Autodesk Inventor part; units mm, degrees
ref_plane "YZ Plane" through (0, 0, 0) normal (1, 0, 0) x (0, 1, 0)
ref_plane "XZ Plane" through (0, 0, 0) normal (0, 1, 0) x (-1, 0, 0)
ref_plane "XY Plane" through (0, 0, 0) normal (0, 0, 1) x (1, 0, 0)
sketch "Sketch1" plane through (0, 0, 0) normal (0, 0, 1) x (1, 0, 0)
  line L0 (0, -3.05) -> (0, 18.3) construction
  line L1 (-3.6, 0) -> (0.6, 0) construction
  line L2 (0, 5) -> (0, 15.25)
  line L3 (0, 15.25) -> (-3, 15.25)
  line L4 (-3, 15.25) -> (-3, 11)
  line L5 (-3, 11) -> (-1, 11)
  line L6 (-1, 11) -> (-1, 5)
  line L7 (-1, 5) -> (0, 5)
  point P0 (0, 0)
  dimension "d0" = 30.5
  dimension "d1" = 10
  dimension "d2" = 22
  dimension "d3" = 1
  dimension "d4" = 3
revolve "Revolution1" add sketch "Sketch1" angle 360 about axis through (-10, 0, 0) along (1, 0, 0)
sketch "Sketch2" plane through (-3, 0, 0) normal (-1, 0, 0) x (0, 0, 1)
  line L0 (0, -21.35) -> (0, 21.35)
  line L1 (-21.35, 0) -> (21.35, 0)
  point P0 (0, 0)
  point P1 (-13, 0)
  dimension "d6" = 13
hole "Hole1" at (-3, 0, -13) direction (1, 0, 0) diameter 2 end through all
mirror "Mirror1" about plane through (0, 0, 0) normal (0, 0, 1) of "Hole1"
properties part number "P119PorteLentilleSouple" material "ABS Plastic"
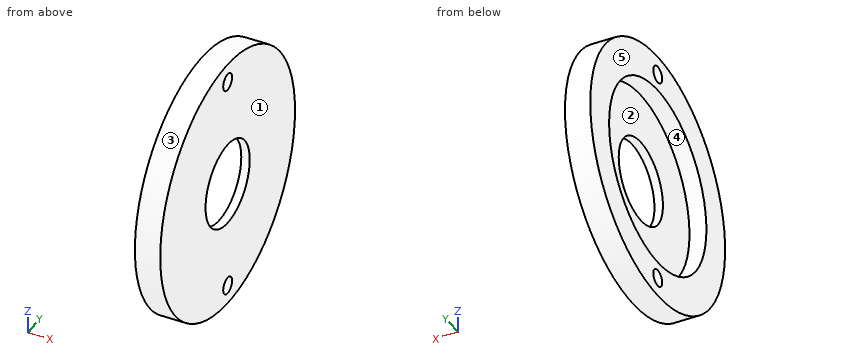
The listing builds one solid part. Answer for the finished solid, in the listing's coordinates (mm). Face numbers are marked on the shaded views. A direction names the side the tool comes from. Give positions to 0.01 mm unless a question says otherwise; leave off trailing zeros. Write each loop counter-clockwise with the first axis right and the second up, starting at its lowest first coordinate (ties: lowest second). Pieces come first, ordered by that corner, then holes. Notation, with made-up numbers: (-28, -19.75) - (20, -19.75) arc R27 cw to (20, 6.25) - close; hole circle Ø2 at (19.5, 13). An arc over 180 degrees is marked (long way). Use a Markdown table: item, result.
1. For a pull along Z with two mould halves and no side action, classify the marked faces 1, 2 and 3 as released by +Z, released by -Z, zero draft, split by the parting line, or undercut.
Values follow:
| item | result |
|---|---|
| face 1 | zero draft |
| face 2 | undercut |
| face 3 | split by the parting line |
2. Section C-C on z = -9 is taken. Write down the section's boundary in (x, y).
Values follow:
| item | result |
|---|---|
| outline | (-3, -12.31) - (0, -12.31) - (0, 12.31) - (-3, 12.31) - (-3, 6.32) - (-1, 6.32) - (-1, -6.32) - (-3, -6.32) - close |
3. Section B-B on z = -13 is taken. Write down the section's boundary in (x, y), plus the area to 3 significant figures.
Values follow:
| item | result |
|---|---|
| outline | (-3, -7.97) - (0, -7.97) - (0, -1) - (-3, -1) - close; (-3, 1) - (0, 1) - (0, 7.97) - (-3, 7.97) - close |
| area | 41.8 mm² |
4. Find the intervals of material crossed by probe 1 along Z at (x, y) = (-2.25, 0); probe 2 along Z at (x, y) = (-0.85, 0); probe 3 along Y at (x, z) = (-1.05, 3), in increasing order. Write a range as from..to.
Values follow:
| item | result |
|---|---|
| probe 1 | z = -15.25..-14, -12..-11, 11..12, 14..15.25 |
| probe 2 | z = -15.25..-14, -12..-5, 5..12, 14..15.25 |
| probe 3 | y = -14.95..-10.58, 10.58..14.95 |
5. A tool of negligible diameter and unlimited length cuts with its end or side. For the marked faces 4 and 5, from which of +Z, -Z, +X, -X, +Y, -Y can it reach the whole face along a straight path? Write none if from no direction.
Values follow:
| item | result |
|---|---|
| face 4 | -X |
| face 5 | +Z, -Z, -X, +Y, -Y |
6. Each of these flat-tipped pins is pushed along its axis until it touches: P1, Ø8, axis at y = 0, z = 0, coming from the +X side; P2, Ø1.5, axis at x = -1.5, z = -4.5, coming from the +Y side; P3, Ø6.5, axis at y = 2.5, z = 4, coming from the -X side. Where does it stop, or does it pass through?
Values follow:
| item | result |
|---|---|
| P1 | passes through |
| P2 | stops at y = 14.78 |
| P3 | stops at x = -1 |
7. Section D-D on x = -1.5 is taken. Write down the section's boundary in (y, z).
Values follow:
| item | result |
|---|---|
| outline | circle Ø30.5 at (0, 0); hole circle Ø22 at (0, 0); hole circle Ø2 at (0, -13); hole circle Ø2 at (0, 13) |
8. Section A-A on y = 0 is taken. Write down the section's boundary in (x, z).
Values follow:
| item | result |
|---|---|
| outline | (-3, -15.25) - (0, -15.25) - (0, -14) - (-3, -14) - close; (-3, -12) - (0, -12) - (0, -5) - (-1, -5) - (-1, -11) - (-3, -11) - close; (-3, 11) - (-1, 11) - (-1, 5) - (0, 5) - (0, 12) - (-3, 12) - close; (-3, 14) - (0, 14) - (0, 15.25) - (-3, 15.25) - close |
